Model file for the job. Use its own axes, mm. Coordinates: 2 decimals unless noted, no trailing zeros. Order: outer loops, then holes, each group sorted by start corner. A loop starts at its lowest first (then second) coordinate and runs counter-clockwise, first axis right, second up. Notation, with made-up numbers: (35.5, 57) -> (94.5, 57) arc R23 ccw to (94.5, 73) -> close; hole circle Ø3 at (-5.75, 3.25). An arc over 180 degrees is marked (long way). Return JSON: item names as keys, results as strings. Group by question number.
1) Cut at C-C (y = 2.25). Write the cut outline in (x, z), and give its area (3 significant figures).
2) Flat gauge pin, fed straight in: pin 1 (3 mm diameter, centred on y = 2.5, z = 12, fed in from +X). Where does the tip first touch, or does it go through?
3) Cut at A-A (x = 0). Write the cut outline in (y, z).
4) Probe line 1 (Z direction, x = 0, y = 5.25); line 2 (X direction, y = 5.25, z = 3.5). List the from-to ranges inside material, lowest first.
5) Pull direction Z, two halves, no side cores. Call faces 1 (the flat face through (18, 4, 0)), 2 (the cylindrical face through (-14.985, 4.563, -0.66)), 3 (the flat face through (-12.654, 3.944, -12.802)): +Z half, -Z half, draft (parallel to the pull), parting line (faces both ways), or undercut.
6) Cut at B-B (z = 0). Write the cut outline in (x, y), and give its area (3 significant figures).
from build123d import *

# Parameters (mm, degrees)
SALIENTE_EXTRUIR1_DEPTH = 9
CROQUIS2_R              = 15
CORTAR_EXTRUIR1_DEPTH   = 10
REDONDEO1_R             = 1


with BuildPart() as part:
    # Croquis1 → Saliente-Extruir1 (new body)
    with BuildSketch(Plane(origin=(0, 0, 0), x_dir=(1, 0, 0), z_dir=(0, 1, 0))):
        Polygon((18, 7.455844123), (7.455844123, 18), (-7.455844123, 18), (-18, 7.455844123), (-18, -7.455844123), (-7.455844123, -18), (7.455844123, -18), (18, -7.455844123), align=None)
    extrude(amount=SALIENTE_EXTRUIR1_DEPTH)

    # Croquis2 → Cortar-Extruir1 (cut, through all)
    with BuildSketch(Plane(origin=(0, 9, 0), x_dir=(1, 0, 0), z_dir=(0, 1, 0))):
        Circle(CROQUIS2_R)
    extrude(amount=-CORTAR_EXTRUIR1_DEPTH, mode=Mode.SUBTRACT)

    # Redondeo1
    redondeo1_edges = [part.edges().sort_by_distance(p)[0] for p in [
        (0, 9, -18),
        (-12.727922061, 9, -12.727922061),
        (-18, 9, 0),
        (-12.727922061, 9, 12.727922061),
        (0, 9, 18),
        (12.727922061, 9, 12.727922061),
        (18, 9, 0),
        (12.727922061, 9, -12.727922061),
    ]]
    fillet(redondeo1_edges, radius=REDONDEO1_R)


solid = part.part
Answers below:
{
 "1": {"outline": "(-18, -7.46) -> (-7.46, -18) -> (7.46, -18) -> (18, -7.46) -> (18, 7.46) -> (7.46, 18) -> (-7.46, 18) -> (-18, 7.46) -> close; hole circle Ø30 at (0, 0)", "area": "367 mm^2"},
 "2": {"pin 1": "stops at x = 14.96"},
 "3": {"outline": "(0, -18) -> (8, -18) arc R1 ccw to (9, -17) -> (9, -15) -> (0, -15) -> close; (0, 15) -> (9, 15) -> (9, 17) arc R1 ccw to (8, 18) -> (0, 18) -> close"},
 "4": {"line 1": "z = -18 to -15, 15 to 18", "line 2": "x = -18 to -14.59, 14.59 to 18"},
 "5": {"face 1": "draft", "face 2": "undercut", "face 3": "-Z half"},
 "6": {"outline": "(-18, 0) -> (-15, 0) -> (-15, 9) -> (-17, 9) arc R1 ccw to (-18, 8) -> close; (15, 0) -> (18, 0) -> (18, 8) arc R1 ccw to (17, 9) -> (15, 9) -> close", "area": "53.6 mm^2"}
}
